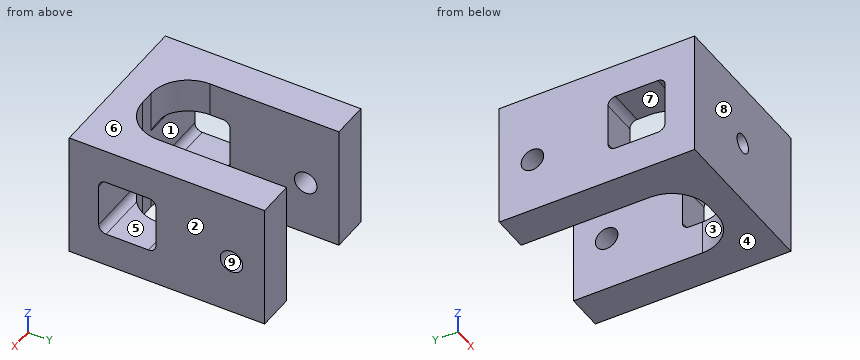
```python
from build123d import *

# Parameters (mm, degrees)
EXTRUDE_1_DEPTH     = 34
SKETCH_2_R          = 2.6
CUT_EXTRUDE_1_DEPTH = 30
SKETCH_3_R          = 3.05
CUT_EXTRUDE_2_DEPTH = 50
SKETCH_8_W          = 15.5
SKETCH_8_H          = 15.5
CUT_EXTRUDE_5_DEPTH = 50
FILLET_4_R          = 2
FILLET_4_2_R        = 10


with BuildPart() as part:
    # Sketch 1 → Extrude 1 (new body)
    with BuildSketch(Plane.XY):
        Polygon((-22, 45.701761355), (-12, 45.701761355), (-12, 0.701761355), (12, 0.701761355), (12, 45.701761355), (22, 45.701761355), (22, -7.298238645), (-22, -7.298238645), align=None)
    extrude(amount=EXTRUDE_1_DEPTH)

    # Sketch 2 → Cut-Extrude 1 (cut, symmetric)
    with BuildSketch(Plane(origin=(0, 0, 0), x_dir=(1, 0, 0), z_dir=(0, 1, 0))):
        with Locations((0, -17)):
            Circle(SKETCH_2_R)
    extrude(amount=CUT_EXTRUDE_1_DEPTH, both=True, mode=Mode.SUBTRACT)

    # Sketch 3 → Cut-Extrude 2 (cut)
    with BuildSketch(Plane.ZY.offset(22)):
        with Locations((15, 36.701761355)):
            Circle(SKETCH_3_R)
    extrude(amount=-CUT_EXTRUDE_2_DEPTH, mode=Mode.SUBTRACT)

    # Sketch 8 → Cut-Extrude 5 (cut)
    with BuildSketch(Plane.ZY.offset(22)):
        with Locations((17, 8.451761355)):
            Rectangle(SKETCH_8_W, SKETCH_8_H)
    extrude(amount=-CUT_EXTRUDE_5_DEPTH, mode=Mode.SUBTRACT)

    # Fillet 4
    fillet_4_edges = [part.edges().sort_by_distance(p)[0] for p in [
        (-17, 16.201761355, 9.25),
        (-17, 16.201761355, 24.75),
        (-17, 0.701761355, 24.75),
        (-17, 0.701761355, 9.25),
        (17, 0.701761355, 9.25),
        (17, 16.201761355, 9.25),
        (17, 0.701761355, 24.75),
        (17, 16.201761355, 24.75),
    ]]
    fillet(fillet_4_edges, radius=FILLET_4_R)

    # Fillet 4 2
    fillet_4_2_edges = [part.edges().sort_by_distance(p)[0] for p in [
        (-12, 0.701761355, 4.625),
        (-12, 0.701761355, 29.375),
        (12, 0.701761355, 29.375),
        (12, 0.701761355, 4.625),
    ]]
    fillet(fillet_4_2_edges, radius=FILLET_4_2_R)


solid = part.part
```
Could you check a few things on this model? Use its own coordinates, in mm. Face numbers are marked on the shaded views. A direction names the side the tool comes from. Round coordinates to 2 decimals unless told otherwise and drop trailing zeros. Loops run counter-clockwise (first coordinate to the right, second up) from the corner with the lowest first, then second, coordinate; pieces in that order, holes last. Notation, with made-up numbers: (6.5, 50.25) - (56.5, 50.25) arc R34 ccw to (56.5, 80.25) - close; hole circle Ø9 at (18, 44.5). An arc over 180 degrees is marked (long way). Use CSV: the item, a comma, the result in double quotes.
Item 1: Will these pins go through, and if not, where does the flat tip stop? pin 1 (8 mm diameter, centred on y = 36.7, z = 15, fed in from -X); pin 2 (10 mm diameter, centred on x = 6, z = 18.5, fed in from +Y).
Here are the results:
pin 1,"stops at x = -22"
pin 2,"stops at y = 0.85"
Item 2: If we section it at C-C on y = 29: List the corners of the cut face in (x, z) for me.
Here are the results:
outline,"(-22, 0) - (-12, 0) - (-12, 34) - (-22, 34) - close; (12, 0) - (22, 0) - (22, 34) - (12, 34) - close"
Item 3: For the marked faces 1, 2, 3, 4 and 5, which set-ups out of +Z, -Z, +X, -X, +Y, -Y let a thin tool reach every point of the face, with its end or its side?
Here are the results:
face 1,"none"
face 2,"+Z, -Z, +X, +Y, -Y"
face 3,"+Z, -Z, +Y"
face 4,"-Z, +X, -X, +Y, -Y"
face 5,"+X, -X"
Item 4: If we section it at B-B on z = 17: List the corners of the cut face in (x, y) for me, then the cut area to 3 significant figures.
Here are the results:
outline,"(-22, -7.3) - (-2.6, -7.3) - (-2.6, 0.7) - (-22, 0.7) - close; (-22, 16.2) - (-12, 16.2) - (-12, 34.4) - (-22, 34.4) - close; (-22, 39) - (-12, 39) - (-12, 45.7) - (-22, 45.7) - close; (2.6, -7.3) - (22, -7.3) - (22, 0.7) - (2.6, 0.7) - close; (12, 16.2) - (22, 16.2) - (22, 34.4) - (12, 34.4) - close; (12, 39) - (22, 39) - (22, 45.7) - (12, 45.7) - close"
area,"808 mm²"
Item 5: If we section it at D-D on y = 10: List the corners of the cut face in (x, z) for me, then the cut area to 3 significant figures.
Here are the results:
outline,"(-22, 0) - (-11.98, 0) - (-11.98, 9.25) - (-22, 9.25) - close; (-22, 24.75) - (-11.98, 24.75) - (-11.98, 34) - (-22, 34) - close; (11.98, 0) - (22, 0) - (22, 9.25) - (11.98, 9.25) - close; (11.98, 24.75) - (22, 24.75) - (22, 34) - (11.98, 34) - close"
area,"371 mm²"
Item 6: If we section it at A-A on x = 0: List the corners of the cut face in (y, z) for me, then the cut area to 3 significant figures.
Here are the results:
outline,"(-7.3, 0) - (0.7, 0) - (0.7, 14.4) - (-7.3, 14.4) - close; (-7.3, 19.6) - (0.7, 19.6) - (0.7, 34) - (-7.3, 34) - close"
area,"230 mm²"
Item 7: I need wall thicknesses on L1, parallel to Y at x = 19.25, z = 15; L2, parallel to X at y = 31, z = 25.5; L3, parallel to X at y = -2, z = 17. Which ranges of each line are inside material? Lowest first, please. Write a range as [from, to].
Here are the results:
L1,"y = [-7.3, 0.7], [16.2, 33.65], [39.75, 45.7]"
L2,"x = [-22, -12], [12, 22]"
L3,"x = [-22, -2.6], [2.6, 22]"
Item 8: If we mould it in two halves opening along Z, with no side actions, what happens to the marked faces 6, 7, 8 and 9? For each: pulls with the +Z half, pulls with the -Z half, needs draft (parallel to the pull), parting line crosses it, or undercut.
Here are the results:
face 6,"pulls with the +Z half"
face 7,"undercut"
face 8,"needs draft"
face 9,"undercut"
